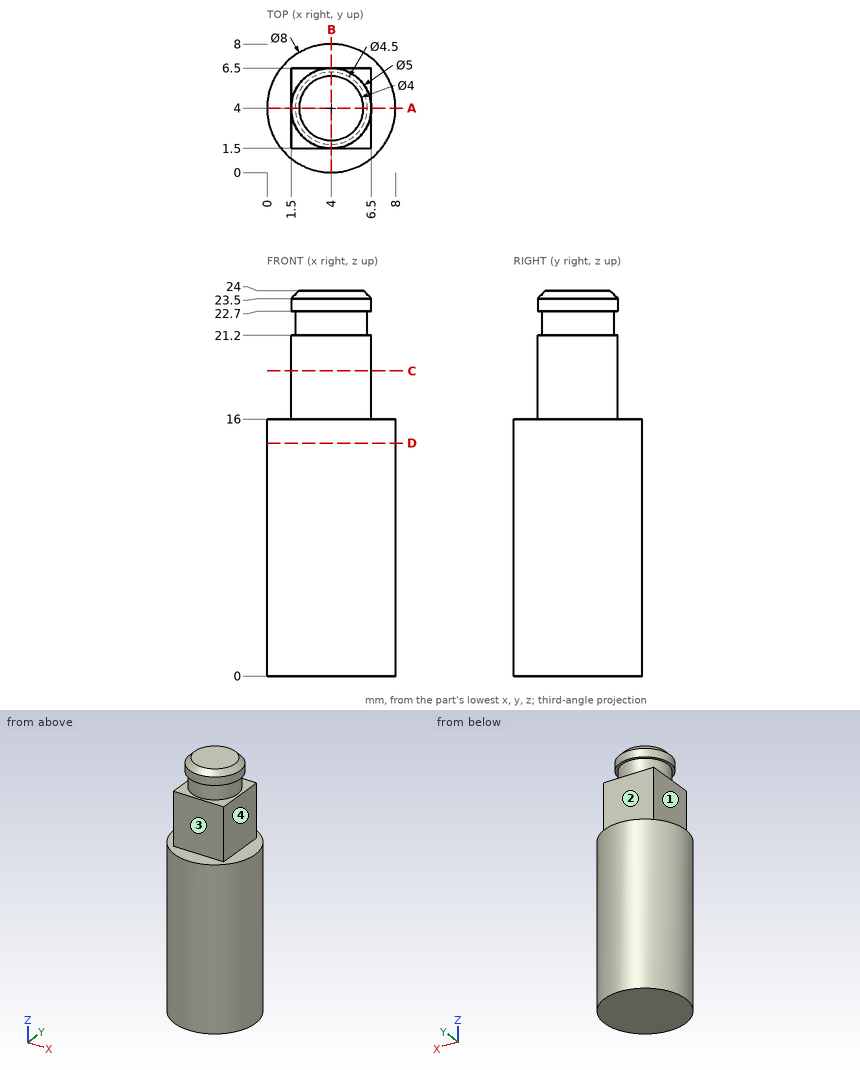
Job drawing, mm, ordinate dimensions from the low corner. One solid piece. A direction names the side the tool comes from. Give positions to 0.01 mm unless a question says otherwise; leave off trailing zeros. Order: outer loops, then holes, each group sorted by start corner. A loop starts at its lowest first (then second) coordinate and runs counter-clockwise, first axis right, second up. Notation, with made-up numbers: (76.5, 18) -> (112.5, 18) arc R35 cw to (112.5, 57) -> close; hole circle Ø3 at (43.25, -18.5). An arc over 180 degrees is marked (long way). Return JSON: item names as keys, results as strings.
Q1. Saw through at A-A (y = 4). Write the cut outline in (x, z).
Working result:
{"outline": "(0, 0) -> (8, 0) -> (8, 16) -> (6.5, 16) -> (6.5, 21.2) -> (6.25, 21.2) -> (6.25, 22.7) -> (6.5, 22.7) -> (6.5, 23.5) -> (6, 24) -> (2, 24) -> (1.5, 23.5) -> (1.5, 22.7) -> (1.75, 22.7) -> (1.75, 21.2) -> (1.5, 21.2) -> (1.5, 16) -> (0, 16) -> close"}
Q2. Drill centre lines: line 1 (Z direction, x = 2.75, y = 0.5); line 2 (X direction, y = 3.5, z = 17.5). Where is each one in solid material? Low to high.
Working result:
{"line 1": "0 to 16", "line 2": "1.5 to 6.5"}
Q3. Saw through at C-C (z = 19). Write the cut outline in (x, y), then the cut area to 3 significant figures.
Working result:
{"outline": "(1.5, 1.5) -> (6.5, 1.5) -> (6.5, 6.5) -> (1.5, 6.5) -> close", "area": "25.0 mm²"}
Q4. Flat gauge pins, fed straight in: pin 1 (1.5 mm diameter, centred on y = 4, z = 19.5, fed in from +X); pin 2 (1 mm diameter, centred on x = 2.5, z = 4, fed in from +Y); pin 3 (2.5 mm diameter, centred on x = 4, z = 18.5, fed in from -Y). Where does each tip first touch, or does it go through?
Working result:
{"pin 1": "x = 6.5", "pin 2": "y = 7.87", "pin 3": "y = 1.5"}
Q5. Which spindle directions (+Z, -Z, +X, -X, +Y, -Y) get a long thin tool onto all of the face, cutting with end or side? Do the marked faces 1, 2, 3 and 4. Say none if no direction does.
Working result:
{"face 1": "+Z, -X, +Y, -Y", "face 2": "+Z, +X, -X, +Y", "face 3": "+Z, +X, -X, -Y", "face 4": "+Z, +X, +Y, -Y"}
Q6. Saw through at D-D (z = 14.5). Write the cut outline in (x, y), then the cut area to 3 significant figures.
Working result:
{"outline": "circle Ø8 at (4, 4)", "area": "50.3 mm²"}
